Could you check a few things on this model? Use its own coordinates, in mm. A direction names the side the tool comes from. Give positions to 0.01 mm unless a question says otherwise; leave off trailing zeros. Order: outer loops, then holes, each group sorted by start corner. A loop starts at its lowest first (then second) coordinate and runs counter-clockwise, first axis right, second up. Notation, with made-up numbers: (3, 79) - (39, 79) arc R22 ccw to (39, 114) - close; hole circle Ø10 at (53.5, -9). An arc over 180 degrees is marked (long way). Put each result on its own line as item: value.
from build123d import *

# Parameters (mm, degrees)
F0_R           = 6.35
F1_DEPTH       = 19.05
F2_SIZE        = 0.762
F3_R           = 9
F4_DEPTH       = 133.35
F5_R           = 11.1125
F6_DEPTH       = 9.525
F7_R           = 0.762
F8_SIZE        = 1.524
F9_W           = 13.2510633147
F9_H           = 4.6713348329
F10_DEPTH      = 11.1135
F10_DEPTH_BACK = 11.1135


with BuildPart() as f1:
    # F0 (on Right) → F1 (new body)
    with BuildSketch(Plane.YZ):
        Circle(F0_R)
    extrude(amount=-F1_DEPTH)

    # F2
    f2_edges = [f1.edges().sort_by_distance(p)[0] for p in [
        (-19.05, -6.35, 0),
    ]]
    chamfer(f2_edges, length=F2_SIZE)

    # F3 (on Right) → F4 (join)
    with BuildSketch(Plane.YZ):
        Circle(F3_R)
    extrude(amount=F4_DEPTH)

    # F5 (on Right) → F6 (join)
    with BuildSketch(Plane.YZ):
        Circle(F5_R)
    extrude(amount=F6_DEPTH)

    # F7
    f7_edges = [f1.edges().sort_by_distance(p)[0] for p in [
        (9.525, -9, 0),
    ]]
    fillet(f7_edges, radius=F7_R)

    # F8
    f8_edges = [f1.edges().sort_by_distance(p)[0] for p in [
        (133.35, -9, 0),
    ]]
    chamfer(f8_edges, length=F8_SIZE)

    # F9 (on Top) → F10 (cut, two sides)
    with BuildSketch(Plane.XY) as f10_sk:
        with Locations((3.6614683426, 11.3356674165)):
            Rectangle(F9_W, F9_H)
        with Locations((3.6614683426, -11.3356674165)):
            Rectangle(F9_W, F9_H)
    extrude(amount=-F10_DEPTH, mode=Mode.SUBTRACT)
    extrude(f10_sk.sketch, amount=F10_DEPTH_BACK, mode=Mode.SUBTRACT)


solid = f1.part
1) If I drill on line 1 (X direction, y = 6.25, z = -8.25) (3 decimals); line 2 (Y direction, x = 123.5, z = 5); line 3 (Z direction, x = 117, y = 0), over which ranges is the centre line in solid material (lowest first)? Write a range as [from, to].
Filled in:
line 1: x = [0, 9.525]
line 2: y = [-7.48, 7.48]
line 3: z = [-9, 9]
2) We'd pull the mould along X, two halves only. Please class faces 1 (the flat face through (9.525, 0, -10)), 2 (the flat face through (5, -9, 0)), 3 (the flat face through (0, -4.1, 5.1)): pulls with the +X half, pulls with the -X half, needs draft (parallel to the pull), parting line crosses it, or undercut.
Filled in:
face 1: pulls with the +X half
face 2: needs draft
face 3: pulls with the -X half
3) Suppose I cut it at B-B, the plane x = 16. List the corners of the cut face in (y, z) for me, and give its area (3 significant figures).
Filled in:
outline: circle Ø18 at (0, 0)
area: 254 mm^2
4) I'm going to push flat-ended pins straight in: pin 1 (5 mm diameter, centred on x = 39.5, y = 0.5, fed in from -Z); pin 2 (3 mm diameter, centred on x = 16, z = -5, fed in from -Y). Where does each tip first touch, or does it pass through?
Filled in:
pin 1: stops at z = -9
pin 2: stops at y = -8.29
5) Which directions (+Z, -Z, +X, -X, +Y, -Y) give clear straight access to the entire face, cutting with the end or side of a thin tool? Please do faces 4 (the cylindrical face through (-9.02, -1.38, -6.2)), 5 (the flat face through (133.35, 0, 0)), 6 (the cylindrical face through (70.206, -1.172, 8.923)), 7 (the flat face through (9.525, 1, 10)).
Filled in:
face 4: -X
face 5: +Z, -Z, +X, +Y, -Y
face 6: +X
face 7: +Z, +X
